```python
from build123d import *

# Parameters (mm, degrees)
SKETCH19_R         = 4
CUT_EXTRUDE3_DEPTH = 25.4


with BuildPart() as part:
    # Sketch1 → Revolve1 (revolve)
    with BuildSketch(Plane.XY):
        with BuildLine():
            Line((0, 0), (0, 11.938))
            Line((0, 11.938), (24.765, 11.938))
            ThreePointArc((24.765, 11.938), (26.561051224, 12.681948776), (27.305, 14.478))
            Line((27.305, 14.478), (27.305, 22.933028409))
            Line((27.305, 22.933028409), (28.104406531, 23.876))
            Line((28.104406531, 23.876), (57.15, 23.876))
            Line((57.15, 23.876), (57.15, 49.2125))
            Line((57.15, 49.2125), (759.206, 49.2125))
            Line((759.206, 49.2125), (759.206, 50.8))
            Line((759.206, 50.8), (771.906, 50.8))
            Line((771.906, 50.8), (771.906, 49.2125))
            Line((771.906, 49.2125), (771.906, 44.1325))
            Line((771.906, 44.1325), (62.23, 44.1325))
            Line((62.23, 44.1325), (62.23, 0))
            Line((62.23, 0), (0, 0))
        make_face()
    revolve(axis=Axis((62.23, 0, 0), (-1, 0, 0)))

    # Sketch16 → Cut-Revolve1 (revolve, cut)
    with BuildSketch(Plane(origin=(0, 0, 0), x_dir=(1, 0, 0), z_dir=(0, 1, 0))):
        Polygon((0, 0), (0, 8.35025), (1.905, 6.556375), (1.905, 0), align=None)
    revolve(axis=Axis((1.905, 0, 0), (-1, 0, 0)), mode=Mode.SUBTRACT)

    # Sketch19 → Cut-Extrude3 (cut)
    with BuildSketch(Plane.ZY.offset(-1.905)):
        Circle(SKETCH19_R)
    extrude(amount=-CUT_EXTRUDE3_DEPTH, mode=Mode.SUBTRACT)

    # Sketch32 → Cut-Revolve6 (revolve, cut)
    with BuildSketch(Plane(origin=(0, 0, 0), x_dir=(1, 0, 0), z_dir=(0, 1, 0)), mode=Mode.PRIVATE) as cut_revolve6_sk:
        Polygon((27.305, 0), (28.575, 0), (27.305, 6.351059428), align=None)
    revolve(cut_revolve6_sk.sketch.rotate(Axis((27.305, 0, 0), (1, 0, 0)), 180), axis=Axis((27.305, 0, 0), (1, 0, 0)), mode=Mode.SUBTRACT)


solid = part.part
```
Here's how the part is built. I have some questions about the finished solid (model axes, mm). A direction names the side the tool comes from. Coordinates: 2 decimals unless noted, no trailing zeros. Order: outer loops, then holes, each group sorted by start corner. A loop starts at its lowest first (then second) coordinate and runs counter-clockwise, first axis right, second up.
1) Imagine slicing it at B-B on y = -37.5. List the corners of the cut face in (x, z) for me, and give its area (3 significant figures).
2) Imagine slicing it at C-C on z = -33. List the corners of the cut face in (x, y) for me.
3) Imagine slicing it at A-A on x = 396. List the corners of the cut face in (y, z) for me (1 decimal), and give its area (3 significant figures).
4) Will these pins go through, and if not, where does the flat tip stop? pin 1 (12 mm diameter, centred on y = -18.5, z = -35, fed in from -X); pin 2 (2 mm diameter, centred on x = 627.5, z = 16.5, fed in from +Y); pin 3 (1.5 mm diameter, centred on x = 100.5, z = -30, fed in from +Y).
5) Which directions (+Z, -Z, +X, -X, +Y, -Y) give clear straight access to the entire face, cutting with the end or side of a thin tool? Please do faces 1 (the face through (27.305, 4.15, -0.09)), 2 (the face through (759.206, 27, -42)), 3 (the face through (771.906, -15, -42)), 4 (the face through (412.1, -32.527, -29.827)).
6) I need wall thicknesses on line 1 (Z direction, x = 544, y = 0); line 2 (Z direction, x = 595, y = 2.5). Which ranges of each line are inside material? Lowest first, please.
7) We'd pull the mould along Z, two halves only. Please class faces 5 (the face through (42.831, -5.176, 23.308)), 6 (the face through (0, 8.13, 2.49)), 7 (the face through (1.905, 3, 3)): +Z half, -Z half, draft (parallel to the pull), parting line (faces both ways), or undercut.
Response values:
1. outline: (57.15, -31.87) - (759.21, -31.87) - (759.21, -34.27) - (771.91, -34.27) - (771.91, -23.27) - (62.23, -23.27) - (62.23, 23.27) - (771.91, 23.27) - (771.91, 34.27) - (759.21, 34.27) - (759.21, 31.87) - (57.15, 31.87) - close
1. area: 12,600 mm2
2. outline: (57.15, -36.51) - (759.21, -36.51) - (759.21, -38.62) - (771.91, -38.62) - (771.91, -29.3) - (62.23, -29.3) - (62.23, 29.3) - (771.91, 29.3) - (771.91, 38.62) - (759.21, 38.62) - (759.21, 36.51) - (57.15, 36.51) - close
3. outline: circle Ø98.4 at (0, 0); hole circle Ø88.3 at (0, 0)
3. area: 1,490 mm2
4. pin 1: stops at x = 57.15
4. pin 2: stops at y = 46.71
4. pin 3: stops at y = 39.58
5. face 1: none
5. face 2: -X
5. face 3: +Z, -Z, +X, +Y, -Y
5. face 4: +X
6. line 1: z = -49.21 to -44.13, 44.13 to 49.21
6. line 2: z = -49.15 to -44.06, 44.06 to 49.15
7. face 5: parting line
7. face 6: draft
7. face 7: undercut
